Geometry: final body of the model. Coordinates: model frame, mm. A direction names the side the tool comes from. Give positions to 0.01 mm unless a question says otherwise; leave off trailing zeros. Write each loop counter-clockwise with the first axis right and the second up, starting at its lowest first coordinate (ties: lowest second). Pieces come first, ordered by that corner, then holes.
Q1. Reachability of faces 4 (the face through (-38, 16.25, 72)), 5 (the face through (-21.5, 11, 61.8)), 6 (the face through (37, -14, 72)) from +Z, -Z, +X, -X, +Y, -Y: full face, straight path, thin tool, end or side. Return the list, or none.
Q2. Pin query (flat end, axial travel): pin 1 (8 mm diameter, centred on y = -3, z = 57, fed in from -X); pin 2 (12 mm diameter, centred on x = 1.5, z = 55.5, fed in from -Y); pin 3 (5 mm diameter, centred on x = 35, z = 76, fed in from +Y); pin 4 (3 mm diameter, centred on x = -22, z = 70.5, fed in from +Y). Return the tip coordinate at first contact, or that it passes through.
Q3. Line query: L1, parallel to Z at x = 26.7, y = 0; L2, parallel to Y at x = 2.5, z = 53; L3, parallel to X at y = -6.5, z = 51. Output: solid intervals per line, ascending.
Q4. Cut plane D-D on z = 76.5. Count the separate pieces of the cut face and the enclosed holes in it, plus the area to 3 significant figures.
Q5. Cut plane A-A on y = 0. Return the cut outline in (x, z), plus the area to 3 significant figures.
Q6. Cut plane C-C on x = 33.5. Return the cut outline in (y, z).
Q7. Draft query along X for faces 1 (the face through (-30, -13, 73)), 2 (the face through (38, -14.25, 72)), 3 (the face through (-27.5, 0, 52)). Return one class per face: pulls with the +X half, pulls with the -X half, needs draft (parallel to the pull), parting line crosses it, or undercut.
Q8. Cut plane B-B on x = 7. Return the cut outline in (y, z).
```python
from build123d import *

# Parameters (mm, degrees)
SKIZZE2_W                       = 55
SKIZZE2_H                       = 30
SKIZZE2_W_2                     = 45
SKIZZE2_H_2                     = 24
AUFSATZ_LINEAR_AUSTRAGEN1_DEPTH = 41
SKIZZE5_W                       = 55
SKIZZE5_H                       = 20
SCHNITT_LINEAR_AUSTRAGEN3_DEPTH = 24
SKIZZE4_R                       = 4
SCHNITT_LINEAR_AUSTRAGEN1_DEPTH = 51
SKIZZE4_3_R                     = 5
SCHNITT_LINEAR_AUSTRAGEN2_DEPTH = 3
SCHNITT_LINEAR_AUSTRAGEN4_DEPTH = 5
SCHNITT_LINEAR_AUSTRAGEN5_DEPTH = 2
AUFSATZ_LINEAR_AUSTRAGEN2_DEPTH = 20
SCHNITT_LINEAR_AUSTRAGEN6_DEPTH = 4
SPIEGELN1_COPY_1_DEPTH          = 5
SPIEGELN1_COPY_2_DEPTH          = 2
SPIEGELN1_COPY_3_DEPTH          = 20
SPIEGELN1_COPY_4_DEPTH          = 4
FASE2_SIZE                      = 2
FASE3_SIZE                      = 4
VERRUNDUNG1_R                   = 2


with BuildPart() as part:
    # Skizze2 → Aufsatz-Linear austragen1 (new body)
    with BuildSketch(Plane.XY.offset(82)):
        Rectangle(SKIZZE2_W, SKIZZE2_H)
        Rectangle(SKIZZE2_W_2, SKIZZE2_H_2, mode=Mode.SUBTRACT)
    extrude(amount=-AUFSATZ_LINEAR_AUSTRAGEN1_DEPTH)

    # Skizze5 → Schnitt-Linear austragen3 (cut)
    with BuildSketch(Plane.XY.offset(82)):
        Rectangle(SKIZZE5_W, SKIZZE5_H)
    extrude(amount=-SCHNITT_LINEAR_AUSTRAGEN3_DEPTH, mode=Mode.SUBTRACT)

    # Skizze4 → Schnitt-Linear austragen1 (cut, through all)
    with BuildSketch(Plane(origin=(22.5, 0, 0), x_dir=(0, 0, -1), z_dir=(1, 0, 0))):
        with Locations((-47.5, 0)):
            Circle(SKIZZE4_R)
    schnitt_linear_austragen1 = extrude(amount=-SCHNITT_LINEAR_AUSTRAGEN1_DEPTH, mode=Mode.SUBTRACT)

    # Skizze4<3> → Schnitt-Linear austragen2 (cut)
    with BuildSketch(Plane(origin=(22.5, 0, 0), x_dir=(0, 0, -1), z_dir=(1, 0, 0))):
        with Locations((-47.5, 0)):
            Circle(SKIZZE4_3_R)
    schnitt_linear_austragen2 = extrude(amount=SCHNITT_LINEAR_AUSTRAGEN2_DEPTH, mode=Mode.SUBTRACT)

    # Skizze6 → Schnitt-Linear austragen4 (cut)
    with BuildSketch(Plane(origin=(0, 15, 0), x_dir=(1, 0, 0), z_dir=(0, 1, 0))):
        with BuildLine():
            Line((26, -61), (26, -79))
            ThreePointArc((26, -79), (25, -80), (24, -79))
            Line((24, -79), (24, -61))
            ThreePointArc((24, -61), (25, -60), (26, -61))
        make_face()
    schnitt_linear_austragen4 = extrude(amount=-SCHNITT_LINEAR_AUSTRAGEN4_DEPTH, mode=Mode.SUBTRACT)

    # Skizze6<3> → Schnitt-Linear austragen5 (cut)
    with BuildSketch(Plane(origin=(0, 15, 0), x_dir=(1, 0, 0), z_dir=(0, 1, 0))):
        with BuildLine():
            Line((23, -61), (23, -79))
            ThreePointArc((23, -79), (25, -81), (27, -79))
            Line((27, -79), (27, -61))
            ThreePointArc((27, -61), (25, -59), (23, -61))
        make_face()
        with BuildLine():
            ThreePointArc((24, -79), (25, -80), (26, -79))
            Line((26, -79), (26, -61))
            ThreePointArc((26, -61), (25, -60), (24, -61))
            Line((24, -61), (24, -79))
        make_face(mode=Mode.SUBTRACT)
        with BuildLine():
            ThreePointArc((25, -59), (26.414213562, -59.585786438), (27, -61))
            Line((27, -61), (27, -79))
            ThreePointArc((27, -79), (25, -81), (23, -79))
            Line((23, -79), (23, -82))
            Line((23, -82), (27.5, -82))
            Line((27.5, -82), (27.5, -59))
            Line((27.5, -59), (25, -59))
        make_face()
    schnitt_linear_austragen5 = extrude(amount=-SCHNITT_LINEAR_AUSTRAGEN5_DEPTH, mode=Mode.SUBTRACT)

    # Skizze8 → Aufsatz-Linear austragen2 (add)
    with BuildSketch(Plane.XY.offset(82)):
        Polygon((27.5, 13), (37, 13), (37, 17.5), (40, 17.5), (40, 10), (27.5, 10), align=None)
    aufsatz_linear_austragen2 = extrude(amount=-AUFSATZ_LINEAR_AUSTRAGEN2_DEPTH)

    # Skizze9 → Schnitt-Linear austragen6 (cut, through all)
    with BuildSketch(Plane.ZY.offset(-37)):
        with BuildLine():
            Line((65, 16.25), (79, 16.25))
            ThreePointArc((79, 16.25), (80, 15.25), (79, 14.25))
            Line((79, 14.25), (65, 14.25))
            ThreePointArc((65, 14.25), (64, 15.25), (65, 16.25))
        make_face()
    schnitt_linear_austragen6 = extrude(amount=-SCHNITT_LINEAR_AUSTRAGEN6_DEPTH, mode=Mode.SUBTRACT)

    # Spiegeln2: Schnitt-Linear austragen4, Schnitt-Linear austragen5, Aufsatz-Linear austragen2, Schnitt-Linear austragen6 across plane
    add(schnitt_linear_austragen4.mirror(Plane.ZX), mode=Mode.SUBTRACT)
    add(schnitt_linear_austragen5.mirror(Plane.ZX), mode=Mode.SUBTRACT)
    add(aufsatz_linear_austragen2.mirror(Plane.ZX))
    add(schnitt_linear_austragen6.mirror(Plane.ZX), mode=Mode.SUBTRACT)

    # Spiegeln1: Schnitt-Linear austragen2, Schnitt-Linear austragen1, Schnitt-Linear austragen4, Schnitt-Linear austragen5, Aufsatz-Linear austragen2, Schnitt-Linear austragen6 across plane
    add(schnitt_linear_austragen2.mirror(Plane(origin=(0, 0, 0), x_dir=(0, 0, 1), z_dir=(1, 0, 0))), mode=Mode.SUBTRACT)
    add(schnitt_linear_austragen1.mirror(Plane(origin=(0, 0, 0), x_dir=(0, 0, 1), z_dir=(1, 0, 0))), mode=Mode.SUBTRACT)
    add(schnitt_linear_austragen4.mirror(Plane(origin=(0, 0, 0), x_dir=(0, 0, 1), z_dir=(1, 0, 0))), mode=Mode.SUBTRACT)
    add(schnitt_linear_austragen5.mirror(Plane(origin=(0, 0, 0), x_dir=(0, 0, 1), z_dir=(1, 0, 0))), mode=Mode.SUBTRACT)
    add(aufsatz_linear_austragen2.mirror(Plane(origin=(0, 0, 0), x_dir=(0, 0, 1), z_dir=(1, 0, 0))))
    add(schnitt_linear_austragen6.mirror(Plane(origin=(0, 0, 0), x_dir=(0, 0, 1), z_dir=(1, 0, 0))), mode=Mode.SUBTRACT)

    # Spiegeln1 copy 1 sketch → Spiegeln1 copy 1 (cut)
    with BuildSketch(Plane(origin=(0, -15, 0), x_dir=(-1, 0, 0), z_dir=(0, -1, 0))):
        with BuildLine():
            Line((26, -61), (26, -79))
            ThreePointArc((26, -79), (25, -80), (24, -79))
            Line((24, -79), (24, -61))
            ThreePointArc((24, -61), (25, -60), (26, -61))
        make_face()
    extrude(amount=-SPIEGELN1_COPY_1_DEPTH, mode=Mode.SUBTRACT)

    # Spiegeln1 copy 2 sketch → Spiegeln1 copy 2 (cut)
    with BuildSketch(Plane(origin=(0, -15, 0), x_dir=(-1, 0, 0), z_dir=(0, -1, 0))):
        with BuildLine():
            Line((23, -61), (23, -79))
            ThreePointArc((23, -79), (25, -81), (27, -79))
            Line((27, -79), (27, -61))
            ThreePointArc((27, -61), (25, -59), (23, -61))
        make_face()
        with BuildLine():
            ThreePointArc((24, -79), (25, -80), (26, -79))
            Line((26, -79), (26, -61))
            ThreePointArc((26, -61), (25, -60), (24, -61))
            Line((24, -61), (24, -79))
        make_face(mode=Mode.SUBTRACT)
        with BuildLine():
            ThreePointArc((25, -59), (26.414213562, -59.585786438), (27, -61))
            Line((27, -61), (27, -79))
            ThreePointArc((27, -79), (25, -81), (23, -79))
            Line((23, -79), (23, -82))
            Line((23, -82), (27.5, -82))
            Line((27.5, -82), (27.5, -59))
            Line((27.5, -59), (25, -59))
        make_face()
    extrude(amount=-SPIEGELN1_COPY_2_DEPTH, mode=Mode.SUBTRACT)

    # Spiegeln1 copy 3 sketch → Spiegeln1 copy 3 (add)
    with BuildSketch(Plane(origin=(0, 0, 82), x_dir=(-1, 0, 0), z_dir=(0, 0, 1))):
        Polygon((27.5, 13), (37, 13), (37, 17.5), (40, 17.5), (40, 10), (27.5, 10), align=None)
    extrude(amount=-SPIEGELN1_COPY_3_DEPTH)

    # Spiegeln1 copy 4 sketch → Spiegeln1 copy 4 (cut, through all)
    with BuildSketch(Plane(origin=(-37, 0, 0), x_dir=(0, 0, 1), z_dir=(1, 0, 0))):
        with BuildLine():
            Line((65, 16.25), (79, 16.25))
            ThreePointArc((79, 16.25), (80, 15.25), (79, 14.25))
            Line((79, 14.25), (65, 14.25))
            ThreePointArc((65, 14.25), (64, 15.25), (65, 16.25))
        make_face()
    extrude(amount=-SPIEGELN1_COPY_4_DEPTH, mode=Mode.SUBTRACT)

    # Fase2
    fase2_edges = [part.edges().sort_by_distance(p)[0] for p in [
        (-22.5, 12, 61.5),
        (-22.5, -12, 61.5),
        (22.5, -12, 61.5),
        (22.5, 12, 61.5),
    ]]
    chamfer(fase2_edges, length=FASE2_SIZE)

    # Fase3
    fase3_edges = [part.edges().sort_by_distance(p)[0] for p in [
        (-33.75, 10, 62),
        (-33.75, -10, 62),
        (33.75, -10, 62),
        (33.75, 10, 62),
    ]]
    chamfer(fase3_edges, length=FASE3_SIZE)

    # Verrundung1
    verrundung1_edges = [part.edges().sort_by_distance(p)[0] for p in [
        (-27.5, 11.5, 64.5),
        (-27.5, -11.5, 64.5),
        (27.5, -11.5, 64.5),
        (27.5, 11.5, 64.5),
    ]]
    fillet(verrundung1_edges, radius=VERRUNDUNG1_R)


solid = part.part
```
Data:
1. face 4: +X, -X
1. face 5: +Z, -Z
1. face 6: +Z, -Z, -Y
2. pin 1: stops at x = -27.5
2. pin 2: stops at y = -15
2. pin 3: stops at y = 17.5
2. pin 4: stops at y = 15
3. L1: z = 41 to 43.5, 51.5 to 58
3. L2: y = -15 to -12, 12 to 15
3. L3: x = -27.5 to -22.5, 22.5 to 27.5
4. separate pieces: 10
4. enclosed holes: 0
4. area: 498 mm2
5. outline: (-27.5, 41) - (-22.5, 41) - (-22.5, 42.5) - (-25.5, 42.5) - (-25.5, 43.5) - (-27.5, 43.5) - close; (-27.5, 51.5) - (-25.5, 51.5) - (-25.5, 52.5) - (-22.5, 52.5) - (-22.5, 58) - (-27.5, 58) - close; (22.5, 41) - (27.5, 41) - (27.5, 43.5) - (25.5, 43.5) - (25.5, 42.5) - (22.5, 42.5) - close; (22.5, 52.5) - (25.5, 52.5) - (25.5, 51.5) - (27.5, 51.5) - (27.5, 58) - (22.5, 58) - close
5. area: 78.0 mm2
6. outline: (-13, 63) - (-10, 66) - (-10, 82) - (-13, 82) - close; (10, 66) - (13, 63) - (13, 82) - (10, 82) - close
7. face 1: undercut
7. face 2: needs draft
7. face 3: pulls with the -X half
8. outline: (-15, 41) - (-12, 41) - (-12, 82) - (-15, 82) - close; (12, 41) - (15, 41) - (15, 82) - (12, 82) - close
